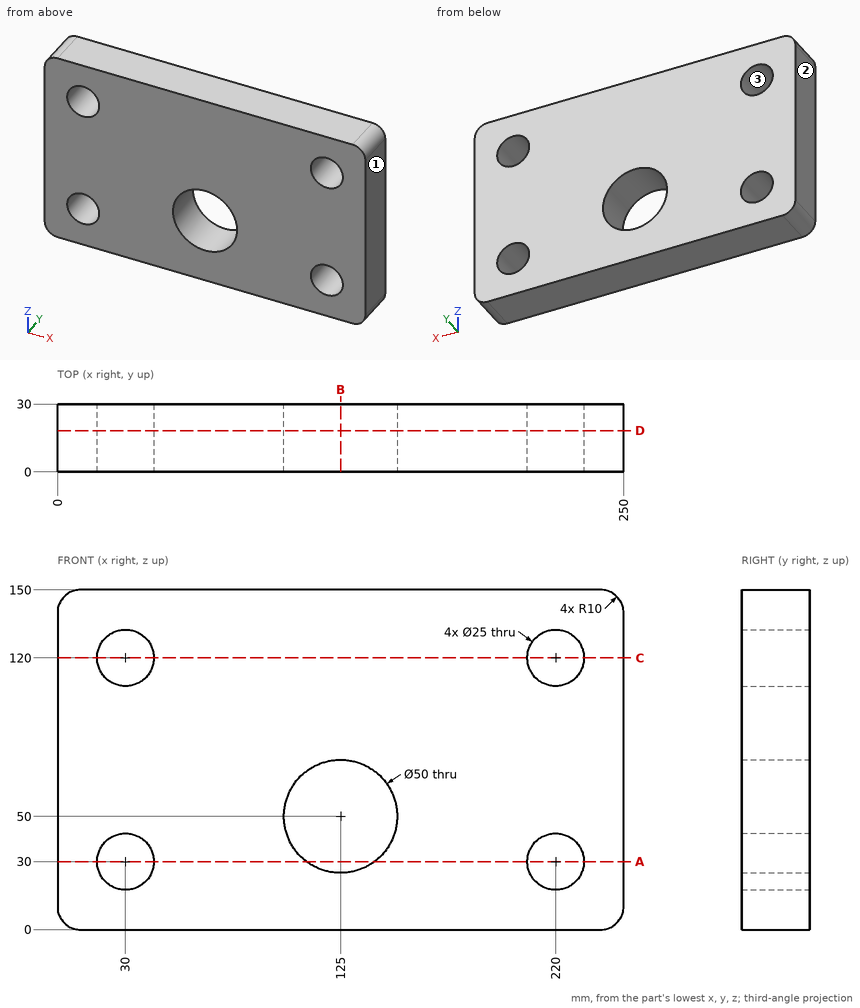
Geometry check sheet. Reference: drawing and pictorial views, mm from the part's lowest x, y, z. Round coordinates to 2 decimals unless told otherwise and drop trailing zeros. Write each loop counter-clockwise with the first axis right and the second up, starting at its lowest first coordinate (ties: lowest second). Pieces come first, ordered by that corner, then holes.
(1) Section check C-C (z = 120). Enter the section's corners in (x, y).
Returned:
outline: (0, 0) - (17.5, 0) - (17.5, 30) - (0, 30) - close; (42.5, 0) - (207.5, 0) - (207.5, 30) - (42.5, 30) - close; (232.5, 0) - (250, 0) - (250, 30) - (232.5, 30) - close
(2) Section check B-B (x = 125). Enter the section's corners in (y, z), plus the area to 3 significant figures.
Returned:
outline: (0, 0) - (30, 0) - (30, 25) - (0, 25) - close; (0, 75) - (30, 75) - (30, 150) - (0, 150) - close
area: 3,000 mm2
(3) Depth check by flat-ended pin: pin 1 Ø8 at (x, y) = (75.5, 21.5) entering from -Z. Enter the tip coordinate at first touch or a pass-through.
Returned:
pin 1: stops at z = 0
(4) Mould release check, pull along X, two halves, no side actions. Record for the marked faces 1, 2 and 3: pulls with the +X half, pulls with the -X half, needs draft (parallel to the pull), parting line crosses it, or undercut.
Returned:
face 1: pulls with the +X half
face 2: pulls with the -X half
face 3: undercut
(5) Section check A-A (z = 30). Enter the section's corners in (x, y).
Returned:
outline: (0, 0) - (17.5, 0) - (17.5, 30) - (0, 30) - close; (42.5, 0) - (110, 0) - (110, 30) - (42.5, 30) - close; (140, 0) - (207.5, 0) - (207.5, 30) - (140, 30) - close; (232.5, 0) - (250, 0) - (250, 30) - (232.5, 30) - close
(6) Section check D-D (y = 18.25). Enter the section's corners in (x, z), plus the area to 3 significant figures.
Returned:
outline: (0, 10) arc R10 ccw to (10, 0) - (240, 0) arc R10 ccw to (250, 10) - (250, 140) arc R10 ccw to (240, 150) - (10, 150) arc R10 ccw to (0, 140) - close; hole circle Ø25 at (30, 30); hole circle Ø25 at (30, 120); hole circle Ø50 at (125, 50); hole circle Ø25 at (220, 30); hole circle Ø25 at (220, 120)
area: 33,500 mm2
(7) Material ranges on line 1 (Z direction, x = 220, y = 8.75); line 2 (X direction, y = 8.5, z = 120); line 3 (Z direction, x = 217, y = 3.75), recorded low to high.
Returned:
line 1: z = 0 to 17.5, 42.5 to 107.5, 132.5 to 150
line 2: x = 0 to 17.5, 42.5 to 207.5, 232.5 to 250
line 3: z = 0 to 17.87, 42.13 to 107.87, 132.13 to 150
